Solid Edge part; units mm, degrees
sketch "Sketch1" plane through (0, 0, 0) normal (0, 0, 1) x (1, 0, 0)
  line L0 (-1, -28) -> (1, -28)
  line L1 (1, -28) -> (1, 28)
  line L2 (1, 28) -> (-1, 28)
  line L3 (-1, 28) -> (-1, -28)
  dimension "D1" = 1
  dimension "D2" = 1
extrude "Protrusion1" add sketch "Sketch1" along normal blind 16
sketch "Sketch2" plane through (0, -28, 8) normal (0, -1, 0) x (0, 0, 1)
  line L0 (-8, -1) -> (-8, -21)
  line L1 (-8, -21) -> (0, -13)
  line L2 (0, -13) -> (8, -21)
  line L3 (8, -21) -> (8, -1)
  dimension "D1" = 8
extrude "Protrusion2" add sketch "Sketch2" against normal up to vertex (56 mm away) material side at (11, -28, 0.05)
sketch "Sketch3" plane through (5, 0, 16) normal (0, 0, 1) x (0, -1, 0)
  line L0 (1.55, 16) -> (-1.55, 16)
  line L1 (-1.55, 16) -> (-1.55, -3)
  line L2 (-1.55, -3) -> (1.55, -3)
  line L3 (1.55, -3) -> (1.55, 16)
  dimension "D1" = 1.55
extrude "Cutout1" cut sketch "Sketch3" against normal through all
sketch "Sketch4" plane through (5, 0, 16) normal (0, 0, 1) x (0, -1, 0)
  line L0 (-28, 16) -> (-23, 16)
  line L1 (-23, 16) -> (-23, -3)
  line L2 (-23, -3) -> (-28, -3)
  line L3 (-28, -3) -> (-28, 16)
extrude "Cutout2" cut sketch "Sketch4" against normal through all
mirror "Mirror1" about plane through (0, 0, 0) normal (0, -1, 0) of "Cutout2"
sketch "Sketch5" plane through (5, 0, 16) normal (0, 0, 1) x (0, -1, 0)
  arc A0 (-1.55, -3) -> (1.55, -3) centre (0, -3) ccw
extrude "Cutout3" cut sketch "Sketch5" against normal through all material side at (0.5, 0, 16)
sketch "Sketch6" plane through (-1, 0, 8) normal (-1, 0, 0) x (0, 0, 1)
  circle A0 centre (0, 12) radius 5.5
  circle A1 centre (0, -12) radius 5.5
extrude "Extrusionsausschnitt_4" cut sketch "Sketch6" against normal blind 3
properties material "Nylon, allgemein"
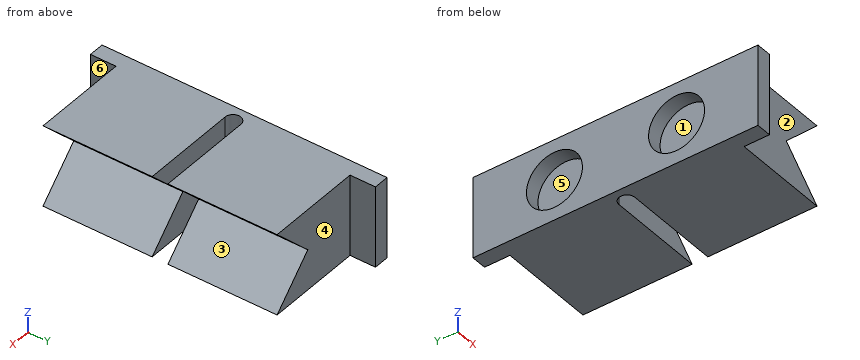
Work out the finished part from the listing and answer in its coordinate system (mm). Face numbers are marked on the shaded views. A direction names the side the tool comes from. Give positions to 0.01 mm unless a question says otherwise; leave off trailing zeros. Loops run counter-clockwise (first coordinate to the right, second up) from the corner with the lowest first, then second, coordinate; pieces in that order, holes last. Notation, with made-up numbers: (-5.5, 73) -> (35.5, 73) arc R27 ccw to (35.5, 104) -> close; hole circle Ø6 at (15, 86). An arc over 180 degrees is marked (long way). Use a Markdown table: item, result. Add a question column.
1) Consider line 1 along Y through (x, z) = (-0.05, 8); line 2 along Y through (x, z) = (7, 9.5); line 3 along Y through (x, z) = (1.2, 8). Determine where each line is inside the solid, lowest interval first.
2) Each of these flat-tipped pins is pushed along its axis until it touches: P1, Ø4, axis at x = 8, z = 10.5, coming from the -Y side; P2, Ø4, axis at y = 16.5, z = 3.5, coming from the +X side; P3, Ø4, axis at y = 24.5, z = 8.5, coming from the +X side. Where does it stop, or does it pass through?
3) The part is cut by section C-C, the plane x = 17. Determine the outline of the cut face in (y, z).
4) Which of the six approach directions +Z, -Z, +X, -X, +Y, -Y give full straight-line access (tool end or side, diameter ignored) to the marked faces 1, 2 and 3?
5) The part is cut by section B-B, the plane y = 12. Determine the outline of the cut face in (x, z).
6) The part is cut by section A-A, the plane x = 1.25. Determine the outline of the cut face in (y, z), plus the area to 3 significant figures.
7) The part is cut by section D-D, the plane x = 11.5. Determine the outline of the cut face in (y, z).
8) For a pull along Y with two mould halves and no side action, classify the marked faces 4, 5 and 6 as +Y half, -Y half, draft (parallel to the pull), parting line (faces both ways), or undercut.
Reported:
| question | item | result |
|---|---|---|
| 1 | line 1 | y = -28 to -17.5, -6.5 to 6.5, 17.5 to 28 |
| 1 | line 2 | y = -23 to -1.55, 1.55 to 23 |
| 1 | line 3 | y = -28 to -17.5, -6.5 to -1.33, 1.33 to 6.5, 17.5 to 28 |
| 2 | P1 | stops at y = -23 |
| 2 | P2 | stops at x = 19.5 |
| 2 | P3 | stops at x = 14.82 |
| 3 | outline | (-23, 0) -> (-1.55, 0) -> (-1.55, 4) -> (-23, 4) -> close; (-23, 12) -> (-1.55, 12) -> (-1.55, 16) -> (-23, 16) -> close; (1.55, 0) -> (23, 0) -> (23, 4) -> (1.55, 4) -> close; (1.55, 12) -> (23, 12) -> (23, 16) -> (1.55, 16) -> close |
| 4 | face 1 | -X |
| 4 | face 2 | +Z, -Z, +X, -Y |
| 4 | face 3 | +X, +Y, -Y |
| 5 | outline | (-1, 0) -> (21, 0) -> (13, 8) -> (21, 16) -> (-1, 16) -> (-1, 13.5) -> (2, 13.5) -> (2, 2.5) -> (-1, 2.5) -> close |
| 6 | outline | (-28, 0) -> (-1.36, 0) -> (-1.36, 16) -> (-28, 16) -> close; (1.36, 0) -> (28, 0) -> (28, 16) -> (1.36, 16) -> close; hole circle Ø11 at (-12, 8); hole circle Ø11 at (12, 8) |
| 6 | area | 663 mm^2 |
| 7 | outline | (-23, 0) -> (-1.55, 0) -> (-1.55, 16) -> (-23, 16) -> close; (1.55, 0) -> (23, 0) -> (23, 16) -> (1.55, 16) -> close |
| 8 | face 4 | +Y half |
| 8 | face 5 | undercut |
| 8 | face 6 | draft |
